Design review of the part built by this model. Coordinates are the model's own, in mm. Face numbers are marked on the shaded views. Give positions to 0.01 mm unless a question says otherwise; leave off trailing zeros. Order: outer loops, then holes, each group sorted by start corner. A loop starts at its lowest first (then second) coordinate and runs counter-clockwise, first axis right, second up. Notation, with made-up numbers: (52, 56.25) - (85, 56.25) arc R14 cw to (85, 70.25) - close; hole circle Ø8 at (43, 61.5). An arc over 180 degrees is marked (long way). Write each question's results on one line, items separated by ' | '. Start each with the question number.
```python
from build123d import *

# Parameters (mm, degrees)
F0_R     = 4.35
F0_R_2   = 3
F1_DEPTH = 5
F2_R     = 10
F2_R_2   = 3
F3_DEPTH = 20
F4_SIZE2 = 6.2
F4_SIZE  = 20
F5_SIZE2 = 5
F5_SIZE  = 19


with BuildPart() as f1:
    # F0 (on Top) → F1 (new body)
    with BuildSketch(Plane.XY):
        Circle(F0_R)
        Circle(F0_R_2, mode=Mode.SUBTRACT)
    extrude(amount=F1_DEPTH)

    # F2 (on face) → F3 (join)
    with BuildSketch(Plane.XY.offset(5)):
        Circle(F2_R)
        Circle(F2_R_2, mode=Mode.SUBTRACT)
    extrude(amount=F3_DEPTH)

    # F4
    f4_edges = [f1.edges().sort_by_distance(p)[0] for p in [
        (-3, 0, 25),
    ]]
    f4_side = f1.faces().sort_by_distance((-3, 0, 12.5))[0]
    chamfer(f4_edges, length=F4_SIZE, length2=F4_SIZE2, reference=f4_side)

    # F5
    f5_edges = [f1.edges().sort_by_distance(p)[0] for p in [
        (-10, 0, 5),
    ]]
    f5_side = f1.faces().sort_by_distance((-10, 0, 15))[0]
    chamfer(f5_edges, length=F5_SIZE, length2=F5_SIZE2, reference=f5_side)


solid = f1.part
```
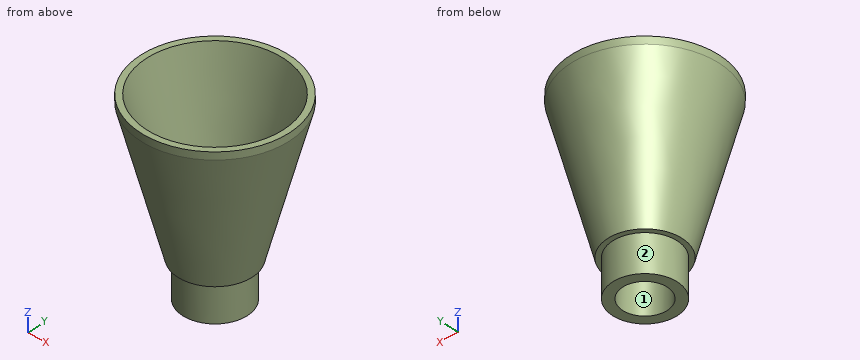
Q1. For line 1 (Y direction, x = 0, z = 3.1); line 2 (Y direction, x = -8, z = 23.5); line 3 (X direction, y = -2.75, z = 17), list the stretches that pass through material, from the lowest coordinate up. Write a range as [from, to].
Q2. Add section D-D (z = 8.75). Give the boundary of the cut face in (x, y) (1 decimal), plus the area to 3 significant figures.
Q3. Insertion check: pin 1 Ø10 at (x, y) = (5, 0) entering from +Z; pin 2 Ø5.5 at (x, y) = (0, 0) entering from -Z; pin 3 Ø12 at (x, z) = (-5, 16) entering from -Y; pin 4 Ø1 at (x, z) = (3, 17.5) entering from +Y. Each pin has a flat end and moves straight along its axis. Give the tip position at first contact, or say it passes through.
Q4. Add section A-A (y = 0). Give the boundary of the cut face in (x, z).
Q5. Draft analysis for pull direction X (two halves, no side actions). For the marked faces 1 and 2, state which applies: pulls with the +X half, pulls with the -X half, needs draft (parallel to the pull), parting line crosses it, or undercut.
Q6. Add section C-C (z = 23.25). Give the boundary of the cut face in (x, y) (1 decimal).
Verdict:
1) line 1: y = [-4.35, -3], [3, 4.35] | line 2: y = [-5.78, -3.51], [3.51, 5.78] | line 3: x = [-7.68, -6.13], [6.13, 7.68]
2) outline: circle Ø12 at (0, 0); hole circle Ø8.3 at (0, 0) | area: 58.2 mm2
3) pin 1: stops at z = 25 | pin 2: passes through | pin 3: stops at y = -9.06 | pin 4: stops at y = 7.95
4) outline: (-10, 24) - (-5, 5) - (-4.35, 5) - (-4.35, 0) - (-3, 0) - (-3, 5) - (-9.2, 25) - (-10, 25) - close; (3, 0) - (4.35, 0) - (4.35, 5) - (5, 5) - (10, 24) - (10, 25) - (9.2, 25) - (3, 5) - close
5) face 1: undercut | face 2: parting line crosses it
6) outline: circle Ø19.6 at (0, 0); hole circle Ø17.3 at (0, 0)
